Autodesk Inventor part; units mm, degrees
ref_plane "housing_to_dummy_XY" through (0, 0, 0) normal (1, 0, 0) x (0, 0, -1)
ref_plane "housing_to_dummy_YZ" through (0, 0, 0) normal (0, 0, -1) x (0, 1, 0)
ref_plane "housing_to_dummy_ZX" through (0, 0, 0) normal (0, 1, 0) x (1, 0, 0)
sketch "Sketch_1" plane through (0, 0, 0) normal (0, 0, 1) x (1, 0, 0)
  line L0 (-25, -20) -> (-25, -30)
  line L1 (-25, -30) -> (25, -30)
  line L2 (25, -30) -> (25, -20)
  line L3 (25, -20) -> (13, -20)
  line L4 (13, -20) -> (13, 14)
  line L5 (13, 14) -> (-13, 14)
  line L6 (-13, 14) -> (-13, -20)
  line L7 (-13, -20) -> (-25, -20)
extrude "Extrusion1" add sketch "Sketch_1" along normal mid plane 10
sketch "Sketch2" plane through (0, 0, 5) normal (0, 0, 1) x (1, 0, 0)
  point P0 (0, 0)
hole "Hole1" at (0, 0, 5) direction (0, 0, -1) diameter 16 depth 10 counterbore diameter 19 counterbore depth 8
sketch "Sketch3" plane through (-25, -30, 5) normal (0, -1, 0) x (1, 0, 0)
  point P0 (6, -5)
hole "Hole2" at (-19, -30, 0) direction (0, 1, 0) diameter 5.5 depth 10
sketch "Sketch4" plane through (-25, -30, 5) normal (0, -1, 0) x (1, 0, 0)
  point P0 (44, -5)
hole "Hole3" at (19, -30, 0) direction (0, 1, 0) diameter 5.5 depth 10
sketch "Sketch_4" plane through (0, 0, 0) normal (1, 0, 0) x (0, 0, -1)
  line L0 (-2, 0) -> (-3.15, 0)
  line L1 (-3.15, 0) -> (-3.15, 10)
  line L2 (-3.15, 10) -> (-2, 10)
  line L3 (-2, 10) -> (-2, 0)
  line L4 (-2, 0) -> (-3.15, 0)
revolve "Revolution1" cut sketch "Sketch_4" angle 360 about axis through (0, 0, 2) along (0, 0, -1)
ref_plane "housing_to_dummy_XY" through (0, 0, 0) normal (1, 0, 0) x (0, 0, -1)
ref_plane "housing_to_dummy_YZ" through (0, 0, 0) normal (0, 0, -1) x (0, 1, 0)
ref_plane "housing_to_dummy_ZX" through (0, 0, 0) normal (0, 1, 0) x (1, 0, 0)
ref_plane "to_bearing_XY" through (0, 0, -3) normal (0, 0, -1) x (1, 0, 0)
ref_plane "to_bearing_YZ" through (0, 0, -3) normal (1, 0, 0) x (0, -1, 0)
ref_plane "to_bearing_ZX" through (0, 0, -3) normal (0, -1, 0) x (0, 0, -1)
ref_plane "to_rring_XY" through (0, 0, 2) normal (0, 0, -1) x (1, 0, 0)
ref_plane "to_rring_YZ" through (0, 0, 2) normal (1, 0, 0) x (0, -1, 0)
ref_plane "to_rring_ZX" through (0, 0, 2) normal (0, -1, 0) x (0, 0, -1)
properties part number "BGHK6800VV-30_h"
The model under review builds one solid part; all positions refer to its coordinate system, in mm. A direction names the side the tool comes from. Round coordinates to 2 decimals unless told otherwise and drop trailing zeros. Write each loop counter-clockwise with the first axis right and the second up, starting at its lowest first coordinate (ties: lowest second). Pieces come first, ordered by that corner, then holes. Notation, with made-up numbers: M 34,58.25 L 84,58.25 A26 ccw 84,93.25 Z; hole C 35,47.25 d5. An arc over 180 degrees is marked long. Answer as CSV lines item,"result". Start each with the question number.
Q1. Consider section A-A, the plane z = 0. Give the boundary of the cut face in (x, y), then the cut area to 3 significant figures.
Q2. Clearance check with flat-ended pins moving along their axes: P1, Ø4, axis at y = 7, z = 2.5, coming from the +X side; P2, Ø4.5, axis at x = 19, z = 0, coming from the +Y side; P3, Ø2, axis at y = 3, z = 2, coming from the -X side. State where each tip first meets the part, or that it passes through.
Q3. Wall thickness on line 1 along X through (y, z) = (-26.5, 0); line 2 along Y through (x, z) = (0, 4.4); line 3 along X through (y, z) = (0, 4.5): over which ranges is each line inside the solid? List them lowest first.
Q4. Consider section C-C, the plane y = 0. Give the boundary of the cut face in (x, z).
Q5. Tool access review of faces 4 (the face through (22, -20, 0)), 5 (the face through (8.43, -4.38, -0.54)), 6 (the face through (-13, -3, 0)): name each direction out of +Z, -Z, +X, -X, +Y, -Y from which nothing blocks a thin tool from reaching the whole face with its end or side.
Q6. Consider section D-D, the plane y = -25.5. Give the boundary of the cut face in (x, z), then the cut area to 3 significant figures.
Q7. The part is to be moulded in two halves that separate along X. For faces 1 (the face through (13, -3, 0)), 2 (the face through (-4, 9, 3.15)), 3 (the face through (0, -13, 5)), say which applies: +X half, -X half, draft (parallel to the pull), parting line (faces both ways), or undercut.
Q8. Consider section B-B, the plane x = 0. Give the boundary of the cut face in (y, z).
Result set:
1,outline,"M -25,-30 L -21.75,-30 L -21.75,-20 L -25,-20 Z; M -16.25,-30 L 16.25,-30 L 16.25,-20 L 13,-20 L 13,14 L -13,14 L -13,-20 L -16.25,-20 Z; M 21.75,-30 L 25,-30 L 25,-20 L 21.75,-20 Z; hole C 0,0 d19"
1,area,"990 mm²"
2,P1,"stops at x = 13"
2,P2,"passes through"
2,P3,"stops at x = -13"
3,line 1,"x = -25 to -21.75, -16.25 to 16.25, 21.75 to 25"
3,line 2,"y = -30 to -9.5, 9.5 to 14"
3,line 3,"x = -13 to -9.5, 9.5 to 13"
4,outline,"M -13,-5 L -8,-5 L -8,-3 L -9.5,-3 L -9.5,2 L -10,2 L -10,3.15 L -9.5,3.15 L -9.5,5 L -13,5 Z; M 8,-5 L 13,-5 L 13,5 L 9.5,5 L 9.5,3.15 L 10,3.15 L 10,2 L 9.5,2 L 9.5,-3 L 8,-3 Z"
5,face 4,"+Z, -Z, +X, +Y"
5,face 5,"+Z"
5,face 6,"+Z, -Z, -X, +Y"
6,outline,"M -25,-5 L 25,-5 L 25,5 L -25,5 Z; hole C -19,0 d5.5; hole C 19,0 d5.5"
6,area,"452 mm²"
7,face 1,"+X half"
7,face 2,"undercut"
7,face 3,"draft"
8,outline,"M -30,-5 L -8,-5 L -8,-3 L -9.5,-3 L -9.5,2 L -10,2 L -10,3.15 L -9.5,3.15 L -9.5,5 L -30,5 Z; M 8,-5 L 14,-5 L 14,5 L 9.5,5 L 9.5,3.15 L 10,3.15 L 10,2 L 9.5,2 L 9.5,-3 L 8,-3 Z"
